Geometry: final body of the model. Coordinates: model frame, mm. Give positions to 0.01 mm unless a question says otherwise; leave off trailing zeros. Write each loop counter-clockwise with the first axis right and the second up, starting at its lowest first coordinate (ties: lowest second). Pieces come first, ordered by that corner, then holes. Notation, with made-up numbers: M 65.5,52 L 97.5,52 A6 ccw 97.5,56 Z; hole C 88.25,-16.75 d10. An arc over 180 degrees is marked long. Use a Markdown table: item, result. Add a question column.
(1) Cut plane C-C (y = 6.5). State how many separate pieces and enclosed holes the cut face has, plus the area to 3 significant figures.
(2) Material intervals for L1, parallel to Z at x = -138.5, y = 7.25; L2, parallel to Z at x = -280, y = 7.25; L3, parallel to Z at x = -30, y = 4.75, sorted ascending.
(3) Cut plane A-A (x = -250). Output: boundary loops of the cut face in (y, z), plus the area to 3 significant figures.
(4) Cut plane B-B (z = -25). Output: boundary loops of the cut face in (x, y), plus the area to 4 significant figures.
Autodesk Inventor part; units mm, degrees
ref_plane "YZ Plane" through (0, 0, 0) normal (1, 0, 0) x (0, 1, 0)
ref_plane "XZ Plane" through (0, 0, 0) normal (0, 1, 0) x (-1, 0, 0)
ref_plane "XY Plane" through (0, 0, 0) normal (0, 0, 1) x (1, 0, 0)
sketch "Skizze1" plane through (0, 0, 0) normal (0, 1, 0) x (-1, 0, 0)
  line L0 (0, 0) -> (275, 0)
  line L1 (275, 0) -> (275, -50)
  line L2 (275, -50) -> (0, -50)
  line L3 (0, -50) -> (0, 0)
  line L4 (275, 0) -> (275, -25)
  line L5 (275, -25) -> (250, -25)
  circle A0 centre (250, -25) radius 15
  line L6 (275, -50) -> (295, -50)
  line L7 (295, -50) -> (295, 0)
  line L8 (295, 0) -> (275, 0)
  dimension "d0" = 275
  dimension "d1" = 50
  dimension "d2" = 25
  dimension "d3" = 30
  dimension "d18" = 20
extrude "Extrusion1" add sketch "Skizze1" along normal blind 9 contours L0 L1 L2 L3
sketch "Skizze2" plane through (0, 9, 0) normal (0, 1, 0) x (1, 0, 0)
  line L0 (0, 0) -> (0, 50)
  line L1 (0, 50) -> (-30, 50)
  line L2 (-30, 50) -> (-30, 35)
  line L3 (0, 0) -> (-55, 0)
  line L4 (-275, 0) -> (0, 0)
  line L5 (-55, 0) -> (-70, 0)
  line L6 (-70, 0) -> (-55, 0)
  line L7 (-55, 0) -> (-55, 15)
  dimension "d6" = 30
  dimension "d7" = 15
  dimension "d8" = 55
  dimension "d9" = 15
  dimension "d10" = 15
hole "Bohrung1" at (-55, 9, -15) at (-30, 9, -35) direction (0, -1, 0) diameter 10 depth 10 tip angle 118
extrude "Extrusion2" add sketch "Skizze1" along normal blind 9 contours L8 L7 L6 L1
sketch "Skizze3" plane through (0, 0, 0) normal (0, -1, 0) x (1, 0, 0)
  line L0 (0, -50) -> (-295, -50)
  line L1 (-295, -50) -> (-280, -50)
  line L2 (-280, -50) -> (-280, -35)
  line L3 (-280, -35) -> (-280, -15)
  line L4 (-280, -15) -> (-280, 0)
  line L5 (-295, 0) -> (0, 0)
  dimension "d21" = 15
  dimension "d22" = 15
  dimension "d23" = 20
hole "Bohrung2" at (-280, 0, -15) at (-280, 0, -35) direction (0, 1, 0) diameter 8 depth 9 tip angle 118
sketch "Skizze4" plane through (0, 0, 0) normal (0, -1, 0) x (1, 0, 0)
  circle A0 centre (-250, -25) radius 15
  line L0 (-250, -25) -> (-223.5, -25)
  line L1 (-223.5, -25) -> (-223.5, -37.5)
  line L2 (-223.5, -37.5) -> (-223.5, -12.5)
  line L3 (-223.5, -12.5) -> (-223.5, -25)
  line L4 (-223.5, -25) -> (-138.5, -25)
  line L5 (-138.5, -25) -> (-138.5, -37.5)
  line L6 (-138.5, -37.5) -> (-138.5, -12.5)
  point P0 (0, 0)
  dimension "d31" = 26.5
  dimension "d32" = 12.5
  dimension "d33" = 25
  dimension "d34" = 85
  dimension "d35" = 12.5
  dimension "d36" = 25
hole "Bohrung3" at (-223.5, 0, -12.5) at (-223.5, 0, -37.5) at (-138.5, 0, -37.5) at (-138.5, 0, -12.5) direction (0, 1, 0) diameter 6 end through all
properties part number "Lagerstuetze" material "Holz (Birke)"
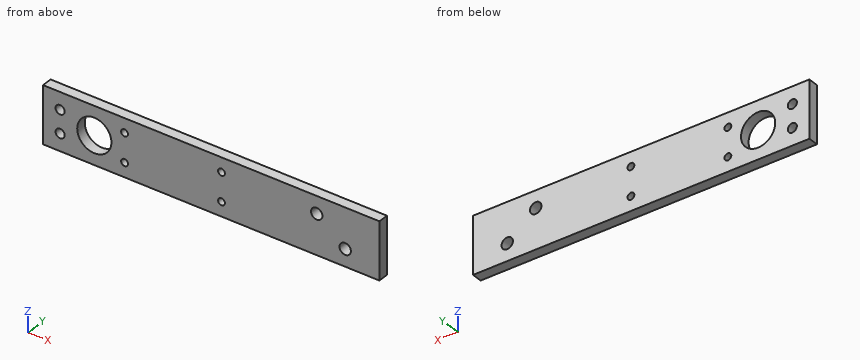
Answer list:
| question | item | result |
|---|---|---|
| 1 | separate pieces | 1 |
| 1 | enclosed holes | 9 |
| 1 | area | 13,700 mm² |
| 2 | L1 | -50 to -40.5, -34.5 to -15.5, -9.5 to 0 |
| 2 | L2 | -50 to -39, -31 to -19, -11 to 0 |
| 2 | L3 | -50 to -40, -30 to 0 |
| 3 | outline | M 0,-50 L 9,-50 L 9,-40 L 0,-40 Z; M 0,-10 L 9,-10 L 9,0 L 0,0 Z |
| 3 | area | 180 mm² |
| 4 | outline | M -295,0 L -265,0 L -265,9 L -295,9 Z; M -235,0 L 0,0 L 0,9 L -235,9 Z |
| 4 | area | 2,385 mm² |
